Verification items for the finished model (mm, model axes). Face numbers are marked on the shaded views. A direction names the side the tool comes from. Give positions to 0.01 mm unless a question says otherwise; leave off trailing zeros. Write each loop counter-clockwise with the first axis right and the second up, starting at its lowest first coordinate (ties: lowest second). Pieces come first, ordered by that corner, then holes.
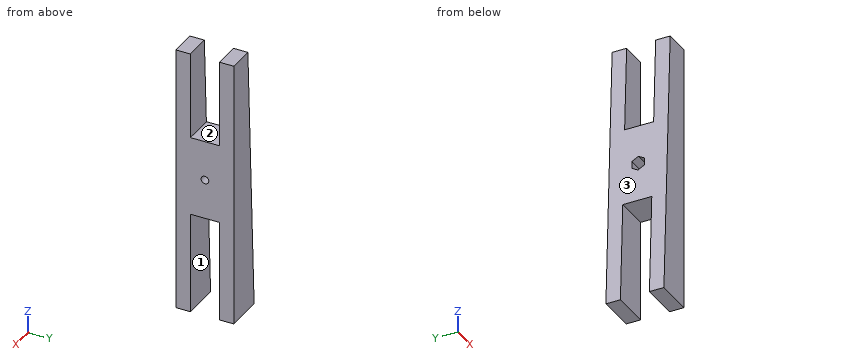
Autodesk Inventor part; units mm, degrees
ref_plane "Work Plane1" through (-20.5163, 50.8, -469.9) normal (1, 0, 0) x (0, 0, -1)
ref_plane "YZ Plane" through (0, 0, 0) normal (1, 0, 0) x (0, 1, 0)
ref_plane "XZ Plane" through (0, 0, 0) normal (0, 1, 0) x (-1, 0, 0)
sketch "Sketch1" plane through (0, 0, 0) normal (0, 1, 0) x (-1, 0, 0)
  line L0 (0, 0) -> (0, -469.9)
  line L1 (0, -469.9) -> (0, -122.0086)
  line L2 (0, -469.9) -> (20.5163, -469.9)
  line L3 (20.5163, -469.9) -> (0, 0)
  dimension "d0" = 469.9
  dimension "d1" = 2.5
extrude "Extrusion1" add sketch "Sketch1" along normal blind 50.8
ref_plane "Work Plane1" through (-20.5163, 50.8, -469.9) normal (1, 0, 0) x (0, 0, -1)
sketch "Sketch2" plane through (0, 0, 0) normal (1, 0, 0) x (0, 0, -1)
  line L0 (0, 0) -> (469.9, 0)
  line L1 (0, 50.8) -> (469.9, 50.8)
  line L2 (0, 0) -> (469.9, 0)
  line L3 (469.9, 0) -> (469.9, 50.8)
  line L4 (469.9, 50.8) -> (0, 50.8)
  line L5 (0, 50.8) -> (0, 0)
extrude "Extrusion2" add sketch "Sketch2" along normal blind 12.7
sketch "Sketch4" plane through (-20.5163, 50.8, -469.9) normal (1, 0, 0) x (0, 0, -1)
  line L0 (0, -50.8) -> (0, 0) construction
  line L1 (0, -25.4) -> (-279.4, -25.4) construction
  line L2 (0, -50.8) -> (-469.9, -50.8) construction
  line L3 (-469.9, -50.8) -> (-469.9, 0) construction
  point P0 (-381, -25.4)
  point P1 (-123.825, -25.4)
  point P2 (-469.9, 0)
  dimension "d16" = 25.4
  dimension "d17" = 88.9
  dimension "d18" = 346.075
hole "Hole2" at (-20.5163, 25.4, -88.9) at (-20.5163, 25.4, -346.075) direction (1, 0, 0) diameter 6.7564 end through all
sketch "Sketch6" plane through (-20.5163, 50.8, -469.9) normal (1, 0, 0) x (0, 0, -1)
  circle A0 centre (-123.825, -25.4) radius 3.3782
  line L0 (-130.2408, -25.4) -> (-127.0329, -19.8438)
  line L1 (-127.0329, -19.8438) -> (-120.6171, -19.8438)
  line L2 (-120.6171, -19.8438) -> (-117.4092, -25.4)
  line L3 (-117.4092, -25.4) -> (-120.6171, -30.9563)
  line L4 (-120.6171, -30.9563) -> (-127.0329, -30.9562)
  line L5 (-127.0329, -30.9562) -> (-130.2408, -25.4)
  circle A1 centre (-381, -25.4) radius 3.3782
  line L6 (-387.4158, -25.4) -> (-384.2079, -19.8438)
  line L7 (-384.2079, -19.8438) -> (-377.7921, -19.8438)
  line L8 (-377.7921, -19.8438) -> (-374.5842, -25.4)
  line L9 (-374.5842, -25.4) -> (-377.7921, -30.9563)
  line L10 (-377.7921, -30.9563) -> (-384.2079, -30.9563)
  line L11 (-384.2079, -30.9563) -> (-387.4158, -25.4)
  line L12 (0, 0) -> (-469.9, 0)
  point P0 (-469.9, -50.8)
  dimension "d26" = 11.1125
extrude "Extrusion3" cut sketch "Sketch6" along normal blind 23.368
ref_plane "Work Plane2" through (-20.5163, 0, -234.95) normal (0, 0, -1) x (-1, 0, 0)
split "Split2" plane through (-20.5163, 0, -234.95) removes the side toward (0, 0, 1)
sketch "Sketch7" plane through (-20.5163, 50.8, -469.9) normal (1, 0, 0) x (0, 0, -1)
  line L0 (-158.75, -38.1) -> (-311.15, -38.1)
  line L1 (-311.15, -38.1) -> (-311.15, -12.7)
  line L2 (-311.15, -12.7) -> (-158.75, -12.7)
  line L3 (-158.75, -12.7) -> (-158.75, -38.1)
  line L4 (-234.95, 0) -> (-234.95, -50.8)
  line L5 (-158.75, -38.1) -> (-311.15, -12.7) construction
  line L6 (-311.15, -38.1) -> (-158.75, -12.7) construction
  line L7 (88.9, -38.1) -> (-88.9, -38.1)
  line L8 (-88.9, -38.1) -> (-88.9, -12.7)
  line L9 (-88.9, -12.7) -> (88.9, -12.7)
  line L10 (88.9, -12.7) -> (88.9, -38.1)
  line L11 (0, -50.8) -> (0, 0)
  line L12 (88.9, -38.1) -> (-88.9, -12.7) construction
  line L13 (-88.9, -38.1) -> (88.9, -12.7) construction
  point P0 (-469.9, -50.8)
  point P1 (-234.95, -25.4)
  point P2 (0, -25.4)
  dimension "d30" = 25.4
  dimension "d31" = 177.8
  dimension "d32" = 152.4
extrude "Extrusion4" cut sketch "Sketch7" along normal through all
equation "\"d0\" = lengthOfFixture"
equation "\"d1\" = cutAngle"
equation "\"d2\" = heightOfJig"
equation "\"d4\" = addedDepthToSupportBolts"
equation "\"d16\" = heightOfBoltHolt"
equation "\"d26\" = hexBoltDiameter"
equation "\"d27\" = depthOfHoleForHexBolt + clearanceForHexbolt"
equation "\"lengthOfFixture\" = 469.9"
equation "\"cutAngle\" = 2.5deg"
equation "\"bottomToFirstHole\" = 88.9"
equation "\"distanceBetweenBolts\" = 257.175"
equation "\"bottomToSecondHole\" = bottomToFirstHole + distanceBetweenBolts"
equation "\"heightOfBoltHolt\" = 25.4"
equation "\"boltSize\" = 6.35"
equation "\"heightOfJig\" = 50.8"
equation "\"addedDepthToSupportBolts\" = 12.7"
equation "\"depthOfHoleForHexBolt\" = 22.86"
equation "\"hexBoltDiameter\" = 11.1125"
equation "\"clearanceForHexbolt\" = 0.508"
equation "\"d29\" = -0.5 * lengthOfFixture"
properties part number "jigForRipCutsB" material "PC/ABS Plastic"
Item 1: Sectioned sample at D-D on z = -280. Record the cut outline in (x, y), then the cut area to 3 significant figures.
Answer key:
outline: (-12.23, 0) - (12.7, 0) - (12.7, 12.7) - (-12.23, 12.7) - close; (-12.23, 38.1) - (12.7, 38.1) - (12.7, 50.8) - (-12.23, 50.8) - close
area: 633 mm2
Item 2: Sectioned sample at C-C on y = 10. Record the cut outline in (x, z), then the cut area to 3 significant figures.
Answer key:
outline: (-20.52, -469.9) - (12.7, -469.9) - (12.7, -234.95) - (-10.26, -234.95) - close
area: 6,600 mm2
Item 3: Set-up check for the marked faces 1, 2 and 3: record each of +Z, -Z, +X, -X, +Y, -Y from which the full face is reachable in a straight line by a thin tool's end or side.
Answer key:
face 1: -Z, +X, -X
face 2: +Z, +X, -X
face 3: +Z, -X, +Y, -Y
Item 4: Sectioned sample at A-A on x = 0.5. Record the cut outline in (y, z).
Answer key:
outline: (0, -469.9) - (12.7, -469.9) - (12.7, -381) - (38.1, -381) - (38.1, -469.9) - (50.8, -469.9) - (50.8, -234.95) - (38.1, -234.95) - (38.1, -311.15) - (12.7, -311.15) - (12.7, -234.95) - (0, -234.95) - close; hole (19.84, -349.28) - (25.4, -352.49) - (30.96, -349.28) - (30.96, -342.87) - (25.4, -339.66) - (19.84, -342.87) - close
Item 5: Sectioned sample at B-B on z = -439. Record the cut outline in (x, y), then the cut area to 3 significant figures.
Answer key:
outline: (-19.17, 0) - (12.7, 0) - (12.7, 12.7) - (-19.17, 12.7) - close; (-19.17, 38.1) - (12.7, 38.1) - (12.7, 50.8) - (-19.17, 50.8) - close
area: 809 mm2
Item 6: Depth check by flat-ended pin: pin 1 (2 mm diameter, centred on x = 7, y = 29, fed in from +Z); pin 2 (6 mm diameter, centred on y = 43, z = -365, fed in from -X); pin 3 (4 mm diameter, centred on y = 33, z = -315, fed in from -X). Enter the tip coordinate at first touch or a pass-through.
Answer key:
pin 1: stops at z = -311.15
pin 2: stops at x = -16.07
pin 3: stops at x = -13.84
Item 7: Scan lines: line 1 along Y through (x, z) = (7, -297.5); line 2 along Z through (x, y) = (5, 25); line 3 along Z through (x, y) = (6.5, 25.4). Record each from-to range of solid material in increasing order.
Answer key:
line 1: y = 0 to 12.7, 38.1 to 50.8
line 2: z = -381 to -349.43, -342.72 to -311.15
line 3: z = -381 to -349.45, -342.7 to -311.15
